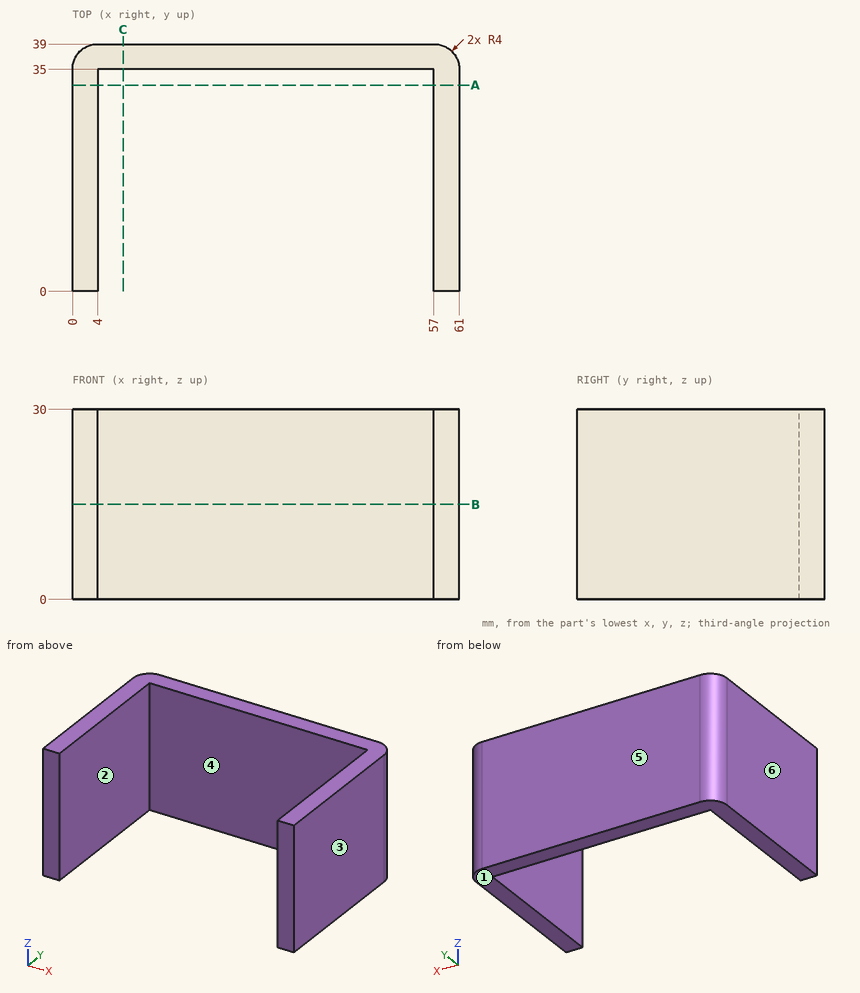
Print and shaded views of the part. All mm, measured from the part's lowest x, y and z. A direction names the side the tool comes from. Coordinates: 2 decimals unless noted, no trailing zeros. Order: outer loops, then holes, each group sorted by start corner. A loop starts at its lowest first (then second) coordinate and runs counter-clockwise, first axis right, second up. Notation, with made-up numbers: (-26, 89.5) - (-1, 89.5) arc R29 cw to (-1, 122.5) - close; hole circle Ø10 at (80, 57). An arc over 180 degrees is marked (long way). Return JSON: item names as keys, results as strings. Group by question number.
Item 1: Pull direction X, two halves, no side cores. Call the marked faces 3, 4, 5 and 6: pulls with the +X half, pulls with the -X half, needs draft (parallel to the pull), parting line crosses it, or undercut.
Item 2: Pin check, flat tip, straight feed: pin 1 (4 mm diameter, centred on x = 46.5, z = 5, fed in from -Y). Stop position of the tip, or through.
Item 3: Cut at A-A (y = 32.5). List the corners of the cut face in (x, z), plus the area to 3 significant figures.
Item 4: Which spindle directions (+Z, -Z, +X, -X, +Y, -Y) get a long thin tool onto all of the face, cutting with end or side? Do the marked faces 1 and 2. Say none if no direction does.
Item 5: Cut at C-C (x = 8). List the corners of the cut face in (y, z), plus the area to 3 significant figures.
Item 6: Cut at B-B (z = 15). List the corners of the cut face in (x, y).
Item 7: Drill centre lines: probe 1 along X at (y, z) = (31.5, 1.5); probe 2 along Y at (x, z) = (12.5, 18); probe 3 along Y at (x, z) = (3, 22.75). Where is each one in solid material? Low to high. Write a range as from..to.
Check values:
{
 "1": {"face 3": "pulls with the +X half", "face 4": "undercut", "face 5": "needs draft", "face 6": "pulls with the -X half"},
 "2": {"pin 1": "stops at y = 35"},
 "3": {"outline": "(0, 0) - (4, 0) - (4, 30) - (0, 30) - close; (57, 0) - (61, 0) - (61, 30) - (57, 30) - close", "area": "240 mm2"},
 "4": {"face 1": "-Z, +X, -X, +Y, -Y", "face 2": "+Z, -Z, -Y"},
 "5": {"outline": "(35, 0) - (39, 0) - (39, 30) - (35, 30) - close", "area": "120 mm2"},
 "6": {"outline": "(0, 0) - (4, 0) - (4, 35) - (57, 35) - (57, 0) - (61, 0) - (61, 35) arc R4 ccw to (57, 39) - (4, 39) arc R4 ccw to (0, 35) - close"},
 "7": {"probe 1": "x = 0..4, 57..61", "probe 2": "y = 35..39", "probe 3": "y = 0..38.87"}
}
